Part model, mm, in its own coordinate system. Face numbers are marked on the shaded views. A direction names the side the tool comes from. Give positions to 0.01 mm unless a question says otherwise; leave off trailing zeros. Write each loop counter-clockwise with the first axis right and the second up, starting at its lowest first coordinate (ties: lowest second). Pieces come first, ordered by that corner, then holes.
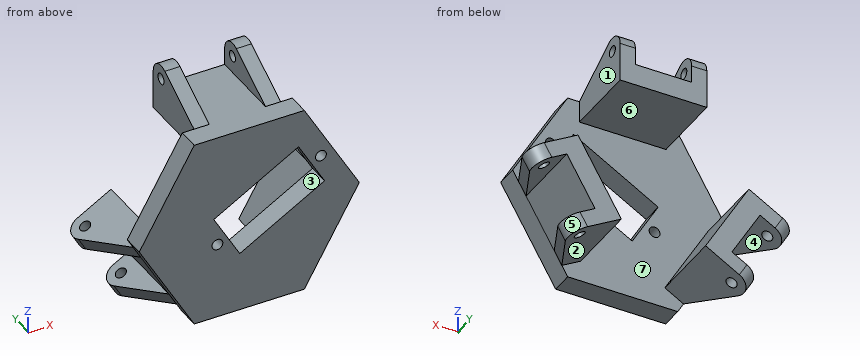
from build123d import *

# Parameters (mm, degrees)
BOSS_EXTRUDE1_DEPTH         = 5
SKETCH4_W                   = 20
SKETCH4_H                   = 5
BOSS_EXTRUDE3_DEPTH         = 17
BOSS_EXTRUDE2_START         = 6.5
SKETCH2_R                   = 1.25
BOSS_EXTRUDE2_DEPTH         = 3.5
CIRPATTERN1_COUNT           = 3
CIRPATTERN1_COPY_1_SKETCH_W = 20
CIRPATTERN1_COPY_1_SKETCH_H = 5
CIRPATTERN1_COPY_1_DEPTH    = 17
CIRPATTERN1_COPY_2_SKETCH_W = 20
CIRPATTERN1_COPY_2_SKETCH_H = 5
CIRPATTERN1_COPY_2_DEPTH    = 17
CIRPATTERN1_START           = 6.5
CIRPATTERN1_COPY_3_SKETCH_R = 1.25
CIRPATTERN1_COPY_3_DEPTH    = 3.5
CIRPATTERN1_COPY_4_SKETCH_R = 1.25
CIRPATTERN1_COPY_4_DEPTH    = 3.5
CUT_EXTRUDE1_REACH          = 47.437
CUT_EXTRUDE2_REACH          = 47.437
SKETCH6_R                   = 1.25


with BuildPart() as part:
    # Sketch1 → Boss-Extrude1 (new body)
    with BuildSketch(Plane(origin=(0, 0, 0), x_dir=(1, 0, 0), z_dir=(0, 1, 0))):
        Polygon((25.403411844, 0), (12.701705922, 22), (-12.701705922, 22), (-25.403411844, 0), (-12.701705922, -22), (12.701705922, -22), align=None)
    extrude(amount=BOSS_EXTRUDE1_DEPTH)

    # Sketch4 → Boss-Extrude3 (add)
    with BuildSketch(Plane(origin=(0, 5, 0), x_dir=(1, 0, 0), z_dir=(0, 1, 0))):
        with Locations((0, -19.5)):
            Rectangle(SKETCH4_W, SKETCH4_H)
    boss_extrude3 = extrude(amount=BOSS_EXTRUDE3_DEPTH)

    # Sketch2 → Boss-Extrude2 (add)
    with BuildSketch(Plane(origin=(0, 0, 0), x_dir=(0, 0, -1), z_dir=(1, 0, 0)).offset(BOSS_EXTRUDE2_START)):
        with BuildLine():
            Line((-22, 22), (-26, 22))
            ThreePointArc((-26, 22), (-28.805149023, 20.391230928), (-28.83316759, 17.157623974))
            Line((-28.83316759, 17.157623974), (-22, 5))
            Line((-22, 5), (-22, 22))
        make_face()
        with Locations(Location((-26, 18.75, 0), (0, 0, 180))):
            Circle(SKETCH2_R, mode=Mode.SUBTRACT)
    boss_extrude2 = extrude(amount=BOSS_EXTRUDE2_DEPTH)

    # Mirror1: Boss-Extrude3, Boss-Extrude2 across plane
    add(boss_extrude3.mirror(Plane(origin=(0, 0, 0), x_dir=(0, 0, 1), z_dir=(1, 0, 0))))
    add(boss_extrude2.mirror(Plane(origin=(0, 0, 0), x_dir=(0, 0, 1), z_dir=(1, 0, 0))))

    # CirPattern1: Boss-Extrude3, Boss-Extrude2 ×3 about axis
    cirpattern1_axis = Axis((0, 0, 0), (0, 1, 0))
    add([boss_extrude3.rotate(cirpattern1_axis, i * 360 / CIRPATTERN1_COUNT) for i in range(1, CIRPATTERN1_COUNT)])
    add([boss_extrude2.rotate(cirpattern1_axis, i * 360 / CIRPATTERN1_COUNT) for i in range(1, CIRPATTERN1_COUNT)])

    # CirPattern1 copy 1 sketch → CirPattern1 copy 1 (add)
    with BuildSketch(Plane(origin=(0, 5, 0), x_dir=(0.4999999999999998, 0, 0.8660254037844387), z_dir=(0, 1, 0))):
        with Locations((0, 19.5)):
            Rectangle(CIRPATTERN1_COPY_1_SKETCH_W, CIRPATTERN1_COPY_1_SKETCH_H)
    extrude(amount=CIRPATTERN1_COPY_1_DEPTH)

    # CirPattern1 copy 2 sketch → CirPattern1 copy 2 (add)
    with BuildSketch(Plane(origin=(0, 5, 0), x_dir=(0.5000000000000004, 0, -0.8660254037844384), z_dir=(0, 1, 0))):
        with Locations((0, 19.5)):
            Rectangle(CIRPATTERN1_COPY_2_SKETCH_W, CIRPATTERN1_COPY_2_SKETCH_H)
    extrude(amount=CIRPATTERN1_COPY_2_DEPTH)

    # CirPattern1 copy 3 sketch → CirPattern1 copy 3 (add)
    with BuildSketch(Plane(origin=(0, 0, 0), x_dir=(-0.8660254037844387, 0, 0.4999999999999998), z_dir=(0.4999999999999998, 0, 0.8660254037844387)).offset(CIRPATTERN1_START)):
        with BuildLine():
            Line((-22, -22), (-26, -22))
            ThreePointArc((-26, -22), (-28.805149023, -20.391230928), (-28.83316759, -17.157623974))
            Line((-28.83316759, -17.157623974), (-22, -5))
            Line((-22, -5), (-22, -22))
        make_face()
        with Locations((-26, -18.75)):
            Circle(CIRPATTERN1_COPY_3_SKETCH_R, mode=Mode.SUBTRACT)
    extrude(amount=CIRPATTERN1_COPY_3_DEPTH)

    # CirPattern1 copy 4 sketch → CirPattern1 copy 4 (add)
    with BuildSketch(Plane(origin=(0, 0, 0), x_dir=(0.8660254037844384, 0, 0.5000000000000004), z_dir=(0.5000000000000004, 0, -0.8660254037844384)).offset(CIRPATTERN1_START)):
        with BuildLine():
            Line((-22, -22), (-26, -22))
            ThreePointArc((-26, -22), (-28.805149023, -20.391230928), (-28.83316759, -17.157623974))
            Line((-28.83316759, -17.157623974), (-22, -5))
            Line((-22, -5), (-22, -22))
        make_face()
        with Locations((-26, -18.75)):
            Circle(CIRPATTERN1_COPY_4_SKETCH_R, mode=Mode.SUBTRACT)
    extrude(amount=CIRPATTERN1_COPY_4_DEPTH)

    # Sketch3 → Cut-Extrude1 (cut, up to next)
    with BuildSketch(Plane(origin=(0, 5, 0), x_dir=(1, 0, 0), z_dir=(0, 1, 0)), mode=Mode.PRIVATE) as cut_extrude1_sk1:
        Polygon((-2.196152423, 8.196152423), (17.376021703, -3.103847577), (11.376021703, -13.496152423), (-8.196152423, -2.196152423), align=None)
    cut_extrude1_tool1 = extrude(cut_extrude1_sk1.sketch, amount=-CUT_EXTRUDE1_REACH, mode=Mode.PRIVATE) & part.part
    add(cut_extrude1_tool1.solids().sort_by_distance((4.589935, 5, 2.65))[0], mode=Mode.SUBTRACT)

    # Sketch6 → Cut-Extrude2 (cut, up to next)
    with BuildSketch(Plane(origin=(0, 5, 0), x_dir=(1, 0, 0), z_dir=(0, 1, 0)), mode=Mode.PRIVATE) as cut_extrude2_sk1:
        with Locations(Location((-7.361215932, 4.25, 0), (0, 0, 270))):
            Circle(SKETCH6_R)
    cut_extrude2_tool1 = extrude(cut_extrude2_sk1.sketch, amount=-CUT_EXTRUDE2_REACH, mode=Mode.PRIVATE) & part.part
    # Sketch6 → Cut-Extrude2 (cut, up to next)
    with BuildSketch(Plane(origin=(0, 5, 0), x_dir=(1, 0, 0), z_dir=(0, 1, 0)), mode=Mode.PRIVATE) as cut_extrude2_sk2:
        with Locations(Location((16.541085212, -9.55, 0), (0, 0, 270))):
            Circle(SKETCH6_R)
    cut_extrude2_tool2 = extrude(cut_extrude2_sk2.sketch, amount=-CUT_EXTRUDE2_REACH, mode=Mode.PRIVATE) & part.part
    add(cut_extrude2_tool1.solids().sort_by_distance((-7.361216, 5, -4.25))[0], mode=Mode.SUBTRACT)
    add(cut_extrude2_tool2.solids().sort_by_distance((16.541085, 5, 9.55))[0], mode=Mode.SUBTRACT)


solid = part.part
1) Mould opens along X. For the marked faces 5, 6 and 7 say: +X half, -X half, draft (parallel to the pull), parting line (faces both ways), or undercut.
Check result:
face 5: +X half
face 6: draft
face 7: undercut
2) Saw through at D-D (y = 6). Write the cut outline in (x, z), and give its area (3 significant figures).
Check result:
outline: (-24.54, -2.62) - (-22.79, -5.65) - (-22.3, -5.37) - (-15.8, -16.63) - (-16.29, -16.91) - (-14.54, -19.94) - (-9.72, -17.16) - (-19.72, 0.16) - close; (-10, 17) - (10, 17) - (10, 22.56) - (6.5, 22.56) - (6.5, 22) - (-6.5, 22) - (-6.5, 22.56) - (-10, 22.56) - close; (9.72, -17.16) - (14.54, -19.94) - (16.29, -16.91) - (15.8, -16.63) - (22.3, -5.37) - (22.79, -5.65) - (24.54, -2.62) - (19.72, 0.16) - close
area: 312 mm2
3) 3-axis set-ups, long thin cutter, end or side, ignore diameter. For the marked faces 1, 2, 3 and 4: which of +Z, -Z, +X, -X, +Y, -Y reach the whole face in a straight line?
Check result:
face 1: +Z, +X, +Y
face 2: -Z, +Y
face 3: +Y, -Y
face 4: -Z, +Y, -Y
4) Saw through at B-B (y = 14). Write the cut outline in (x, z), and give its area (3 significant figures).
Check result:
outline: (-28.43, -4.87) - (-26.68, -7.9) - (-22.3, -5.37) - (-15.8, -16.63) - (-20.18, -19.16) - (-18.43, -22.19) - (-9.72, -17.16) - (-19.72, 0.16) - close; (-10, 17) - (10, 17) - (10, 27.06) - (6.5, 27.06) - (6.5, 22) - (-6.5, 22) - (-6.5, 27.06) - (-10, 27.06) - close; (9.72, -17.16) - (18.43, -22.19) - (20.18, -19.16) - (15.8, -16.63) - (22.3, -5.37) - (26.68, -7.9) - (28.43, -4.87) - (19.72, 0.16) - close
area: 406 mm2
5) Saw through at A-A (x = -4). Write the cut outline in (y, z).
Check result:
outline: (0, -22) - (5, -22) - (5, -5.07) - (0, -5.07) - close; (0, 4.62) - (5, 4.62) - (5, 17) - (22, 17) - (22, 22) - (0, 22) - close
6) Flat gauge pins, fed straight in: P1, Ø1, axis at x = 8, y = 10, coming from the -Z side; P2, Ø3.5, axis at y = 15.5, z = 27, coming from the -X side; P3, Ø1.5, axis at x = 2, y = 5.5, coming from the +Z side. Where does each tip first touch, or does it go through?
Check result:
P1: stops at z = 17
P2: stops at x = -10
P3: stops at z = 22
7) Drill centre lines: L1, parallel to X at y = 12.5, z = 24.5; L2, parallel to Z at x = 7.55, y = 18.75; L3, parallel to Z at x = 2.5, y = 10.5. Where is each one in solid material? Low to high.
Check result:
L1: x = -10 to -6.5, 6.5 to 10
L2: z = 17 to 24.75, 27.25 to 29.25
L3: z = 17 to 22
8) Saw through at C-C (z = 9.55). Write the cut outline in (x, y), and give its area (3 significant figures).
Check result:
outline: (-19.89, 0) - (4.54, 0) - (4.54, 5) - (-19.89, 5) - close; (13.65, 0) - (15.29, 0) - (15.29, 5) - (13.65, 5) - close; (17.79, 0) - (19.89, 0) - (19.89, 5) - (17.79, 5) - close
area: 141 mm2
